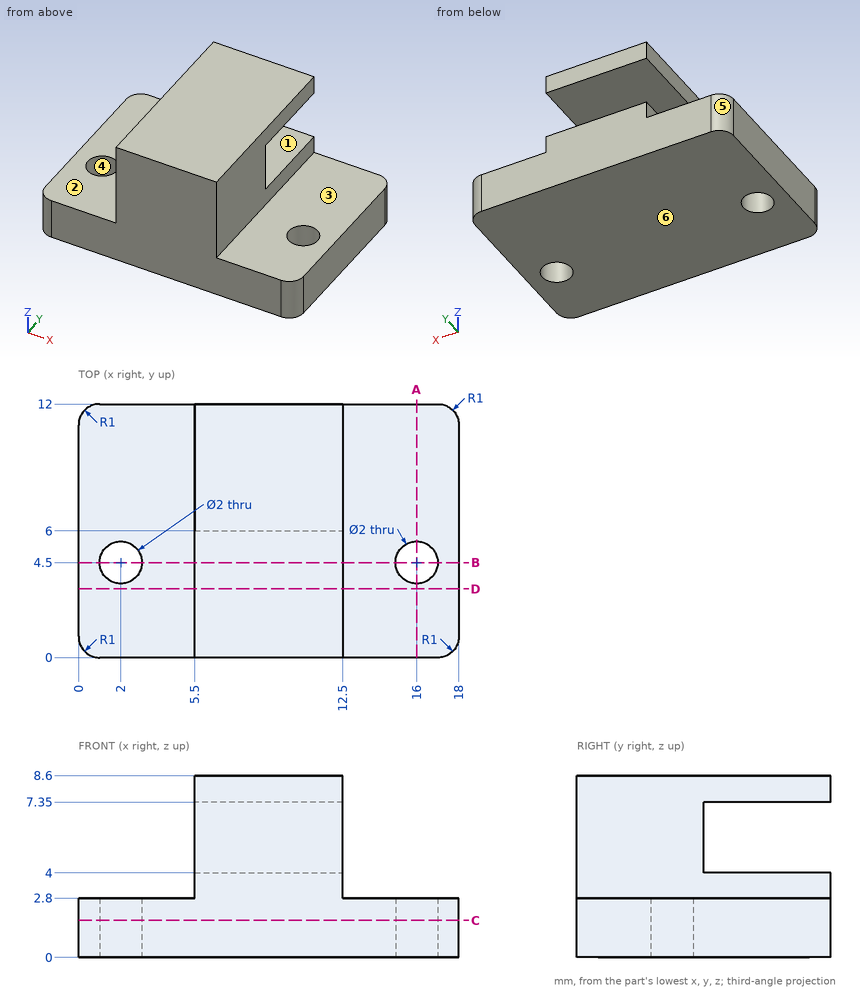
Source: three-view drawing plus pictorial views. Frame: mm from the lowest corner of the part. A direction names the side the tool comes from. Give positions to 0.01 mm unless a question says otherwise; leave off trailing zeros. Order: outer loops, then holes, each group sorted by start corner. A loop starts at its lowest first (then second) coordinate and runs counter-clockwise, first axis right, second up.
1. Section D-D on y = 3.25. Return the cut outline in (x, z), and give its area (3 significant figures).
Derived:
outline: (0, 0) - (18, 0) - (18, 2.8) - (12.5, 2.8) - (12.5, 8.6) - (5.5, 8.6) - (5.5, 2.8) - (0, 2.8) - close
area: 91.0 mm2
2. Mould query, pull axis Y, two halves, no side actions, for the marked faces 4, 5 and 6. Classes: released by +Y, released by -Y, zero draft, split by the parting line, or undercut.
Derived:
face 4: undercut
face 5: released by +Y
face 6: zero draft
3. Reachability of the marked faces 1, 2 and 3 from +Z, -Z, +X, -X, +Y, -Y: full face, straight path, thin tool, end or side. Return the list, or none.
Derived:
face 1: +X, -X, +Y
face 2: +Z, -X, +Y, -Y
face 3: +Z, +X, +Y, -Y
4. Material intervals for L1, parallel to X at y = 4.5, z = 1.4; L2, parallel to Y at x = 2, z = 1.55; L3, parallel to X at y = 4, z = 2.75, sorted ascending.
Derived:
L1: x = 0 to 1, 3 to 15, 17 to 18
L2: y = 0 to 3.5, 5.5 to 12
L3: x = 0 to 1.13, 2.87 to 15.13, 16.87 to 18
5. Pin query (flat end, axial travel): pin 1 (1.7 mm diameter, centred on y = 3.5, z = 7, fed in from -X); pin 2 (1.2 mm diameter, centred on x = 16, y = 4.5, fed in from -Z); pin 3 (4.5 mm diameter, centred on x = 2.5, y = 4.5, fed in from +Z). Return the tip coordinate at first contact, or that it passes through.
Derived:
pin 1: stops at x = 5.5
pin 2: passes through
pin 3: stops at z = 2.8
6. Section B-B on y = 4.5. Return the cut outline in (x, z), and give its area (3 significant figures).
Derived:
outline: (0, 0) - (1, 0) - (1, 2.8) - (0, 2.8) - close; (3, 0) - (15, 0) - (15, 2.8) - (12.5, 2.8) - (12.5, 8.6) - (5.5, 8.6) - (5.5, 2.8) - (3, 2.8) - close; (17, 0) - (18, 0) - (18, 2.8) - (17, 2.8) - close
area: 79.8 mm2
7. Section A-A on x = 16. Return the cut outline in (y, z), and give its area (3 significant figures).
Derived:
outline: (0, 0) - (3.5, 0) - (3.5, 2.8) - (0, 2.8) - close; (5.5, 0) - (12, 0) - (12, 2.8) - (5.5, 2.8) - close
area: 28.0 mm2
8. Section C-C on z = 1.75. Return the cut outline in (x, y).
Derived:
outline: (0, 1) arc R1 ccw to (1, 0) - (17, 0) arc R1 ccw to (18, 1) - (18, 11) arc R1 ccw to (17, 12) - (1, 12) arc R1 ccw to (0, 11) - close; hole circle Ø2 at (2, 4.5); hole circle Ø2 at (16, 4.5)
